Source: three-view drawing plus pictorial views. Frame: mm from the lowest corner of the part. A direction names the side the tool comes from. Give positions to 0.01 mm unless a question says otherwise; leave off trailing zeros. Order: outer loops, then holes, each group sorted by start corner. A loop starts at its lowest first (then second) coordinate and runs counter-clockwise, first axis right, second up. Notation, with made-up numbers: (60.5, 34) -> (92.5, 34) arc R19 cw to (92.5, 66) -> close; hole circle Ø2 at (31.5, 57). An arc over 180 degrees is marked (long way). Answer in a Markdown table with one row per item. Add a question column.
Q1. Line query: line 1 along X through (y, z) = (4, 32); line 2 along Z through (x, y) = (35, 2.75); line 3 along X through (y, z) = (7.5, 41) (1 decimal). Output: solid intervals per line, ascending. Write a range as from..to.
Q2. Set-up query: the marked faces 4 and 5. Return all of +Z, -Z, +X, -X, +Y, -Y with unobstructed straight access to the full face (end or side cutting, diameter ignored); none if empty.
Q3. Pull-direction query (Z, two-part tool) for the marked faces 1, 2 and 3; classes: +Z half, -Z half, draft (parallel to the pull), parting line (faces both ways), or undercut.
Q4. Cut plane C-C on z = 17.5. Return the cut outline in (x, y).
Q5. Cut plane A-A on x = 5.08. Return the cut outline in (y, z).
Q6. Cut plane D-D on x = 18. Return the cut outline in (y, z).
Q7. Contact query for a flat-ended pin moving along its axis: P1, Ø4.5, axis at x = 29, y = 4, coming from the -Z side. Output: stop coordinate, or through.
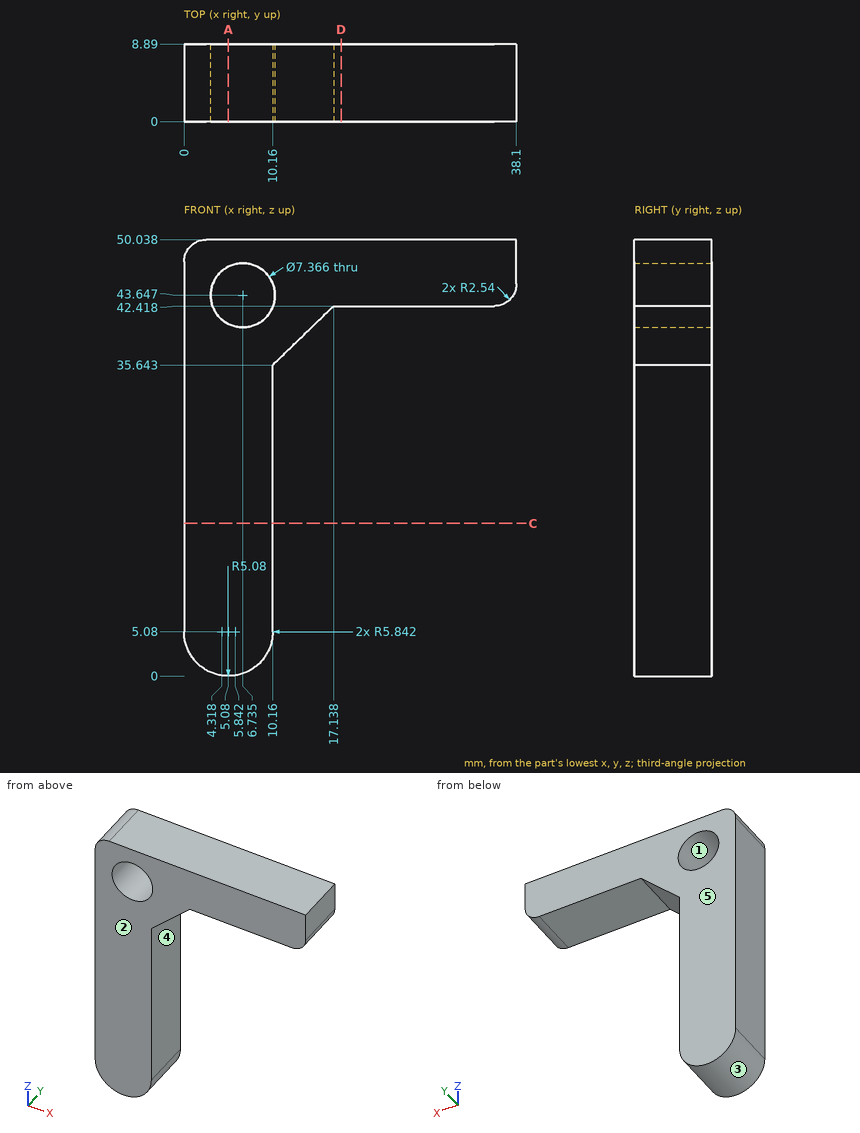
Completed:
| question | item | result |
|---|---|---|
| 1 | line 1 | x = 0..10.16 |
| 1 | line 2 | z = 42.42..50.04 |
| 1 | line 3 | x = 0..4.2, 9.3..15.7 |
| 2 | face 4 | -Z, +X, +Y, -Y |
| 2 | face 5 | +Z, -Z, +X, -X, +Y |
| 3 | face 1 | undercut |
| 3 | face 2 | draft |
| 3 | face 3 | -Z half |
| 4 | outline | (0, 0) -> (10.16, 0) -> (10.16, 8.89) -> (0, 8.89) -> close |
| 5 | outline | (0, 0) -> (8.89, 0) -> (8.89, 40.36) -> (0, 40.36) -> close; (0, 46.94) -> (8.89, 46.94) -> (8.89, 50.04) -> (0, 50.04) -> close |
| 6 | outline | (0, 42.42) -> (8.89, 42.42) -> (8.89, 50.04) -> (0, 50.04) -> close |
| 7 | P1 | stops at z = 42.42 |
